Geometry: see drawing. Coordinates: mm, zero at the bounding-box minimum. A direction names the side the tool comes from. Coordinates: 2 decimals unless noted, no trailing zeros. Write each loop counter-clockwise with the first axis right and the second up, starting at its lowest first coordinate (ties: lowest second). Pieces come first, ordered by that corner, then holes.
1) Set-up query: the marked faces 1, 2 and 3. Return all of +Z, -Z, +X, -X, +Y, -Y with unobstructed straight access to the full face (end or side cutting, diameter ignored); none if empty.
2) Section query C-C (y = 12.5). Output: boundary loops of the cut face in (x, z).
3) Line query: L1, parallel to X at y = 6.5, z = 0.95. Output: solid intervals per line, ascending.
4) Pin query (flat end, axial travel): pin 1 Ø1.4 at (x, z) = (1, 1) entering from -Y; pin 2 Ø1 at (y, z) = (10.5, 0.5) entering from +X; pin 3 Ø1.5 at (y, z) = (10.5, 1.5) entering from -X. Return the tip coordinate at first contact, or that it passes through.
5) Draft query along Y for the marked faces 4, 5 and 6. Return one class per face: pulls with the +Y half, pulls with the -Y half, needs draft (parallel to the pull), parting line crosses it, or undercut.
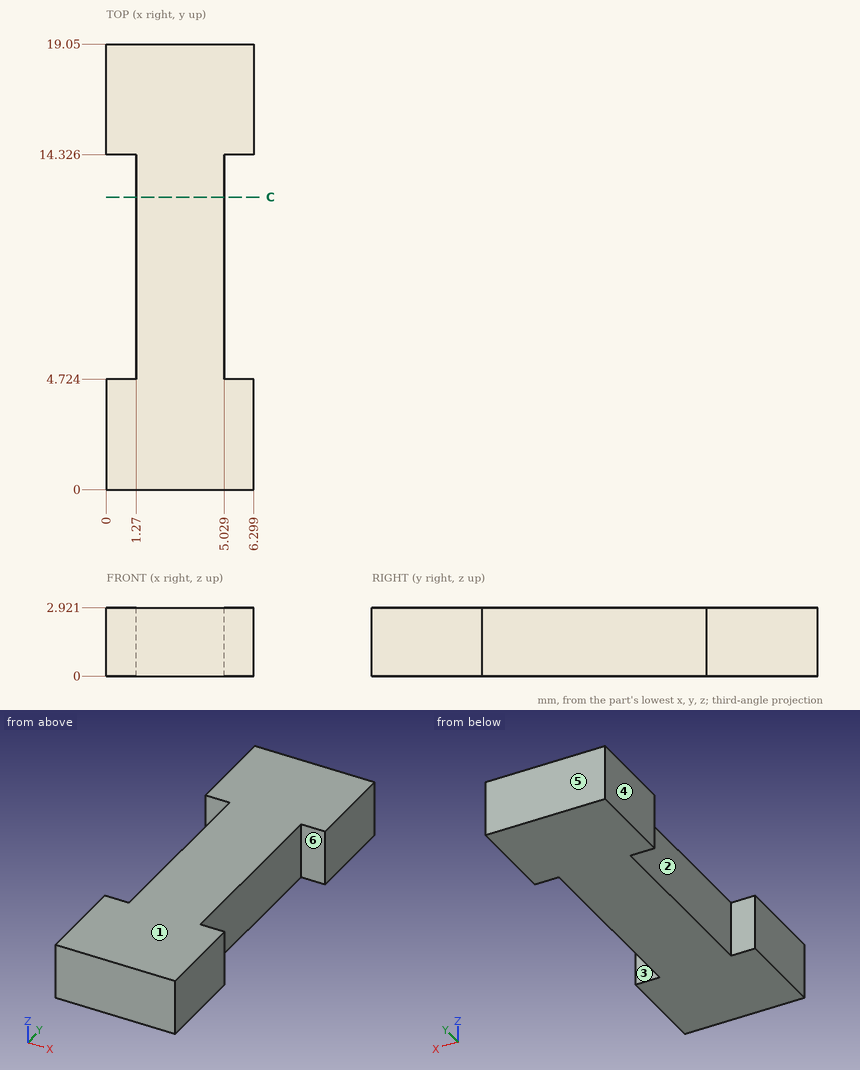
Answer:
1. face 1: +Z, +X, -X, +Y, -Y
1. face 2: +Z, -Z, -X
1. face 3: +Z, -Z, +X
2. outline: (1.27, 0) - (5.03, 0) - (5.03, 2.92) - (1.27, 2.92) - close
3. L1: x = 1.27 to 5.03
4. pin 1: stops at y = 0
4. pin 2: stops at x = 5.03
4. pin 3: stops at x = 1.27
5. face 4: needs draft
5. face 5: pulls with the +Y half
5. face 6: undercut
